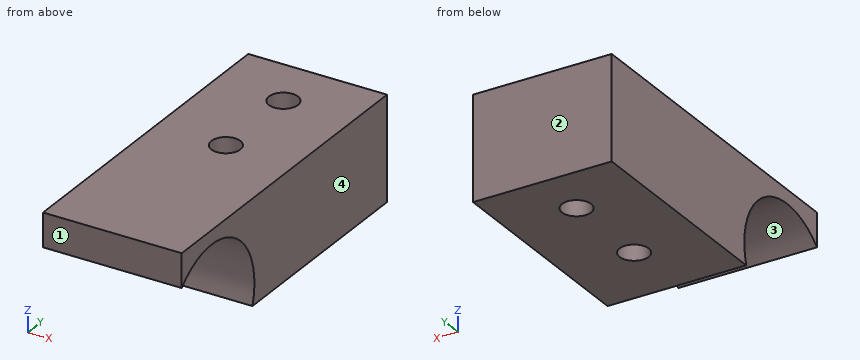
```python
from build123d import *

# Parameters (mm, degrees)
F0_W     = 20
F0_H     = 48
F1_DEPTH = 15
F2_R     = 10
F3_DEPTH = 25
F4_R     = 2.1
F5_DEPTH = 25


with BuildPart() as f1:
    # F0 (on Top) → F1 (new body)
    with BuildSketch(Plane.XY):
        with Locations((-13.931248, 14.507082)):
            Rectangle(F0_W, F0_H)
    extrude(amount=F1_DEPTH)

    # F2 (on Right) → F3 (cut)
    with BuildSketch(Plane.YZ):
        with Locations((-2.492918, 3)):
            Circle(F2_R)
    extrude(amount=-F3_DEPTH, mode=Mode.SUBTRACT)

    # F4 (on face) → F5 (cut)
    with BuildSketch(Plane(origin=(0, 0, 0), x_dir=(1, 0, 0), z_dir=(0, 0, -1))):
        with Locations((-13.931248, -30.507082)):
            Circle(F4_R)
        with Locations((-13.931248, -17.046474)):
            Circle(F4_R)
    extrude(amount=-F5_DEPTH, mode=Mode.SUBTRACT)


solid = f1.part
```
Could you check a few things on this model? Use its own coordinates, in mm. Face numbers are marked on the shaded views. Coordinates: 2 decimals unless noted, no trailing zeros. Write each loop counter-clockwise with the first axis right and the second up, starting at its lowest first coordinate (ties: lowest second). Pieces come first, ordered by that corner, then holes. Notation, with made-up numbers: (-17, 47.5) -> (-4, 47.5) arc R29 ccw to (-4, 74.5) -> close; hole circle Ø1 at (42.25, 1.5). An arc over 180 degrees is marked (long way). Write item = value, one per line. Start each with the question number.
(1) Will these pins go through, and if not, where does the flat tip stop? pin 1 (4 mm diameter, centred on x = -13.93, y = 30.51, fed in from -Z); pin 2 (10 mm diameter, centred on x = -16, y = 6, fed in from -Z).
(2) I want a section at D-D (x = -20.5). Please give me the cut outline in (y, z), plus the area to 3 significant figures.
(3) I want a section at B-B (x = -13.5). Please give me the cut outline in (y, z), plus the area to 3 significant figures.
(4) I want a section at A-A (z = 12.5). Please give me the cut outline in (x, y).
(5) We'd pull the mould along Y, two halves only. Please class the marked faces 1, 2, 3 and 4: released by +Y, released by -Y, zero draft, split by the parting line, or undercut.
(6) I need wall thicknesses on line 1 (Y direction, x = -12.75, z = 1.25); line 2 (Y direction, x = -12.75, z = 5.75); line 3 (Y direction, x = -11.5, z = 11.75). Which ranges of each line are inside material? Lowest first, please. Write a range as [from, to].
(7) I want a section at C-C (y = 15.5). Please give me the cut outline in (x, z).
Result set:
q1.pin_1 = through
q1.pin_2 = 0
q2.outline = (-9.49, 10.14) arc R10 cw to (7.05, 0) -> (38.51, 0) -> (38.51, 15) -> (-9.49, 15) -> close
q2.area = 527 mm2
q3.outline = (-9.49, 10.14) arc R10 cw to (7.05, 0) -> (14.99, 0) -> (14.99, 15) -> (-9.49, 15) -> close; (19.1, 0) -> (28.45, 0) -> (28.45, 15) -> (19.1, 15) -> close; (32.56, 0) -> (38.51, 0) -> (38.51, 15) -> (32.56, 15) -> close
q3.area = 404 mm2
q4.outline = (-23.93, -9.49) -> (-3.93, -9.49) -> (-3.93, -5.62) -> (-23.93, -5.62) -> close; (-23.93, 0.63) -> (-3.93, 0.63) -> (-3.93, 38.51) -> (-23.93, 38.51) -> close; hole circle Ø4.2 at (-13.93, 17.05); hole circle Ø4.2 at (-13.93, 30.51)
q5.face_1 = released by -Y
q5.face_2 = released by +Y
q5.face_3 = undercut
q5.face_4 = zero draft
q6.line_1 = [7.35, 15.31], [18.78, 28.77], [32.24, 38.51]
q6.line_2 = [7.12, 15.31], [18.78, 28.77], [32.24, 38.51]
q6.line_3 = [-9.49, -7.33], [2.35, 38.51]
q7.outline = (-23.93, 0) -> (-15.35, 0) -> (-15.35, 15) -> (-23.93, 15) -> close; (-12.51, 0) -> (-3.93, 0) -> (-3.93, 15) -> (-12.51, 15) -> close
